from build123d import *

# Parameters (mm, degrees)
SKETCH2_W           = 152.4
SKETCH2_H           = 152.4
SKETCH2_R           = 3.2004
SKETCH2_R_2         = 3.556
SKETCH2_R_3         = 2
BOSS_EXTRUDE1_DEPTH = 4.7625


with BuildPart() as part:
    # Sketch2 → Boss-Extrude1 (new body)
    with BuildSketch(Plane(origin=(0, 0, 0), x_dir=(1, 0, 0), z_dir=(0, 1, 0))):
        with Locations((76.2, 50.8)):
            Rectangle(SKETCH2_W, SKETCH2_H)
        with Locations((139.419367389, 14.8828125)):
            Circle(SKETCH2_R, mode=Mode.SUBTRACT)
        with Locations((139.419367389, 86.7171875)):
            Circle(SKETCH2_R, mode=Mode.SUBTRACT)
        with Locations((142.24, 116.84)):
            Circle(SKETCH2_R_2, mode=Mode.SUBTRACT)
        with Locations((10.16, 116.84)):
            Circle(SKETCH2_R_2, mode=Mode.SUBTRACT)
        with Locations((10.16, -15.24)):
            Circle(SKETCH2_R_2, mode=Mode.SUBTRACT)
        with Locations((142.24, -15.24)):
            Circle(SKETCH2_R_2, mode=Mode.SUBTRACT)
        with Locations((12.451545477, 30.80004)):
            Circle(SKETCH2_R_3, mode=Mode.SUBTRACT)
        with Locations((43.904269028, 30.80004)):
            Circle(SKETCH2_R_3, mode=Mode.SUBTRACT)
        with Locations((43.904269028, 70.79996)):
            Circle(SKETCH2_R_3, mode=Mode.SUBTRACT)
        with Locations((12.451545477, 70.79996)):
            Circle(SKETCH2_R_3, mode=Mode.SUBTRACT)
    extrude(amount=BOSS_EXTRUDE1_DEPTH)


solid = part.part
Could you check a few things on this model? Use its own coordinates, in mm. Give positions to 0.01 mm unless a question says otherwise; leave off trailing zeros. Loops run counter-clockwise (first coordinate to the right, second up) from the corner with the lowest first, then second, coordinate; pieces in that order, holes last. Notation, with made-up numbers: (65.25, 3.5) -> (74.25, 3.5) arc R14 cw to (74.25, 27.5) -> close; hole circle Ø9 at (71.25, 45). An arc over 180 degrees is marked (long way). Return JSON: item names as keys, results as strings.
Item 1: We'd pull the mould along Z, two halves only. Please class faces 1 (the cylindrical face through (41.906, 2.348, -30.888)), 2 (the flat face through (75, 2, -127)), 3 (the flat face through (0, 2, -50)): +Z half, -Z half, draft (parallel to the pull), parting line (faces both ways), or undercut.
Geometry results:
{"face 1": "undercut", "face 2": "-Z half", "face 3": "draft"}
Item 2: If we section it at A-A on z = -116.84: List the corners of the cut face in (x, y) for me, plus the area to 3 significant figures.
Geometry results:
{"outline": "(0, 0) -> (6.6, 0) -> (6.6, 4.76) -> (0, 4.76) -> close; (13.72, 0) -> (138.68, 0) -> (138.68, 4.76) -> (13.72, 4.76) -> close; (145.8, 0) -> (152.4, 0) -> (152.4, 4.76) -> (145.8, 4.76) -> close", "area": "658 mm²"}
Item 3: I need wall thicknesses on L1, parallel to X at y = 2.6, z = 15.24; L2, parallel to Z at x = 8, y = 2.3; L3, parallel to Z at x = 142.24, y = 1.1. Which ranges of each line are inside material? Lowest first, please. Write a range as from..to.
Geometry results:
{"L1": "x = 0..6.6, 13.72..138.68, 145.8..152.4", "L2": "z = -127..-119.66, -114.02..12.42, 18.06..25.4", "L3": "z = -127..-120.4, -113.28..-88.23, -85.21..-16.39, -13.37..11.68, 18.8..25.4"}
